from build123d import *

# Parameters (mm, degrees)
SKETCH1_W           = 4.5
SKETCH1_H           = 76
SKETCH2_W           = 19
SKETCH2_H           = 19
BOSS_EXTRUDE1_DEPTH = 6
FILLET4_R           = 1
SKETCH7_OUTSIDE_W   = 58.258
SKETCH7_OUTSIDE_H   = 58.258
SKETCH7_OUTSIDE_R   = 9.5
CUT_EXTRUDE1_DEPTH  = 10
CUT_EXTRUDE1_DRAFT  = -45


with BuildPart() as part:
    # Sketch1 → Revolve1 (revolve)
    with BuildSketch(Plane.XY):
        with Locations((2.25, -38)):
            Rectangle(SKETCH1_W, SKETCH1_H)
    revolve(axis=Axis((4.5, 0, 0), (0, -1, 0)))

    # Sketch2 → Boss-Extrude1 (add)
    with BuildSketch(Plane(origin=(0, 0, 0), x_dir=(1, 0, 0), z_dir=(0, 1, 0))):
        with Locations((4.5, 0)):
            Rectangle(SKETCH2_W, SKETCH2_H)
    extrude(amount=BOSS_EXTRUDE1_DEPTH)

    # Fillet4
    fillet4_edges = [part.edges().sort_by_distance(p)[0] for p in [
        (9, -76, 0),
    ]]
    fillet(fillet4_edges, radius=FILLET4_R)


with BuildPart() as cut_extrude1_tool:
    # Sketch7 outside → Cut-Extrude1 (with draft: the straight prism first)
    with BuildSketch(Plane(origin=(0, 6, 0), x_dir=(1, 0, 0), z_dir=(0, 1, 0))):
        with Locations((4.5, 0)):
            Rectangle(SKETCH7_OUTSIDE_W, SKETCH7_OUTSIDE_H)
        with Locations((4.5, 0)):
            Circle(SKETCH7_OUTSIDE_R, mode=Mode.SUBTRACT)
    extrude(amount=-CUT_EXTRUDE1_DEPTH)
    # Cut-Extrude1: the draft: its side faces are tilted about the plane it starts from
    cut_extrude1_sides = [cut_extrude1_tool.faces().sort_by_distance(p)[0] for p in [
        (4.5, 1, 29.129),
        (33.629, 1, 0),
        (4.5, 1, -29.129),
        (-24.629, 1, 0),
        (-5, 1, 0),
    ]]
    draft(cut_extrude1_sides, Plane(origin=(0, 6, 0), x_dir=(1, 0, 0), z_dir=(0, 1, 0)), CUT_EXTRUDE1_DRAFT)


with BuildPart() as part_1:
    add(part.part)

    # Cut-Extrude1: cut by cut_extrude1_tool
    add(cut_extrude1_tool.part, mode=Mode.SUBTRACT)


solid = part_1.part
The model under review builds one solid part; all positions refer to its coordinate system, in mm. A direction names the side the tool comes from. Round coordinates to 2 decimals unless told otherwise and drop trailing zeros. Write each loop counter-clockwise with the first axis right and the second up, starting at its lowest first coordinate (ties: lowest second). Pieces come first, ordered by that corner, then holes. Notation, with made-up numbers: (41.25, 7) - (61.25, 7) arc R28 ccw to (61.25, 37) - close; hole circle Ø3 at (64.5, 61.5). An arc over 180 degrees is marked (long way). One line per item, written item: value. Start each with the question number.
1. Machinability: for faces 4 (the face through (4, 2, -9.5)), 5 (the face through (5.09, -36.98, -4.46)), which of the approach directions +Z, -Z, +X, -X, +Y, -Y give a long, thin tool a straight path to every point of the face, cutting with its end or side? Answer none if there is none.
2. Clearance check with flat-ended pins moving along their axes: P1, Ø1.5, axis at y = -64, z = 0.5, coming from the +X side; P2, Ø10, axis at x = 1, z = -7.5, coming from the -Y side; P3, Ø3, axis at x = 9.5, y = -43, coming from the -Z side. State where each tip first meets the part, or that it passes through.
3. Consider section A-A on y = -6. Write out the cut boundary in (x, z), and give its area (3 significant figures).
4. The part is to be moulded in two halves that separate along Y. For faces 1 (the face through (-2.908, 5.062, 7.354)), 2 (the face through (4, 2, 9.5)), 3 (the face through (0, 0, -2)), say which applies: released by +Y, released by -Y, zero draft, split by the parting line, or undercut.
5. To check wall thickness, follow L1, parallel to X at y = -43, z = 0; L2, parallel to Z at x = 4.25, y = -25; L3, parallel to Y at x = -3.5, z = 3.75. State the ranges of each line that lie inside material, in increasing order. Write a range as from..to.
Checks:
1. face 4: -Z, +X, -X, +Y, -Y
1. face 5: -Y
2. P1: stops at x = 9
2. P2: stops at y = -76
2. P3: stops at z = -2.83
3. outline: circle Ø9 at (4.5, 0)
3. area: 63.6 mm^2
4. face 1: released by +Y
4. face 2: zero draft
4. face 3: released by -Y
5. L1: x = 0..9
5. L2: z = -4.49..4.49
5. L3: y = 0..6
